Answer from the drawing. Dimensions are ordinates in mm from the lowest x, y and z of the part. A direction names the side the tool comes from. Round coordinates to 2 decimals unless told otherwise and drop trailing zeros. Write each loop counter-clockwise with the first axis right and the second up, starting at its lowest first coordinate (ties: lowest second). Pieces come first, ordered by that corner, then holes.
1. A flat-ended cylindrical pin translates along its axis: pin 1 Ø6 at (x, z) = (57, 7.5) entering from +Y. Find the tip coordinate at first contact, or state that the pin passes through.
2. Find section A-A (z = 6.5). Write down the section's boundary in (x, y), and give its area (3 significant figures).
3. Straight lines are drawn through the part: probe 1 along Z at (x, y) = (86, 8.5); probe 2 along Y at (x, z) = (99.4, 12.3); probe 3 along Z at (x, y) = (79, 0.7). For each, find the intervals that lie inside material, in ascending order.
4. Find section C-C (x = 79). Write down the section's boundary in (y, z).
5. A tool of negligible diameter and unlimited length cuts with its end or side. For the marked faces 1 and 2, from which of +Z, -Z, +X, -X, +Y, -Y can it reach the whole face along a straight path? Write none if from no direction.
6. Find section B-B (y = 7.75). Write down the section's boundary in (x, z), and give its area (3 significant figures).
7. Find section D-D (x = 92). Write down the section's boundary in (y, z), and give its area (3 significant figures).
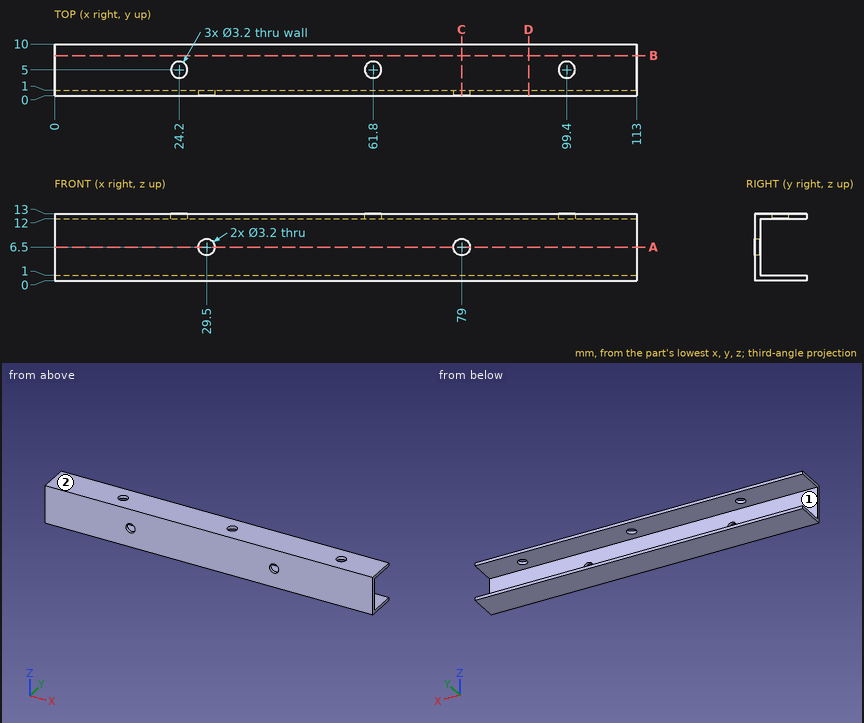
Worked answers:
1. pin 1: stops at y = 1
2. outline: (0, 0) - (27.9, 0) - (27.9, 1) - (0, 1) - close; (31.1, 0) - (77.4, 0) - (77.4, 1) - (31.1, 1) - close; (80.6, 0) - (113, 0) - (113, 1) - (80.6, 1) - close
2. area: 107 mm2
3. probe 1: z = 0 to 1, 12 to 13
3. probe 2: y = 0 to 3.4, 6.6 to 10
3. probe 3: z = 0 to 4.9, 8.1 to 13
4. outline: (0, 0) - (10, 0) - (10, 1) - (1, 1) - (1, 4.9) - (0, 4.9) - close; (0, 8.1) - (1, 8.1) - (1, 12) - (10, 12) - (10, 13) - (0, 13) - close
5. face 1: +X, -X, +Y
5. face 2: +Z, +X, -X, +Y, -Y
6. outline: (0, 0) - (113, 0) - (113, 1) - (0, 1) - close; (0, 12) - (113, 12) - (113, 13) - (0, 13) - close
6. area: 226 mm2
7. outline: (0, 0) - (10, 0) - (10, 1) - (1, 1) - (1, 12) - (10, 12) - (10, 13) - (0, 13) - close
7. area: 31.0 mm2
